Verification items for the finished model (mm, model axes). A direction names the side the tool comes from. Give positions to 0.01 mm unless a question says otherwise; leave off trailing zeros. Order: outer loops, then holes, each group sorted by start corner. A loop starts at its lowest first (then second) coordinate and runs counter-clockwise, first axis right, second up.
(1) Sectioned sample at C-C on x = 1.25. Record the cut outline in (y, z), plus the area to 3 significant figures.
(2) Gauge pin test, flat ends, axial feed: pin 1 (5 mm diameter, centred on x = 2, y = 0.5, fed in from -Z); pin 2 (2 mm diameter, centred on x = 8.5, z = 4.5, fed in from -Y); pin 3 (2 mm diameter, centred on x = 1.5, y = -10, fed in from +Z); pin 4 (7 mm diameter, centred on x = 0, y = 0, fed in from +Z). Record the tip position at first contact, or that the pin passes through.
(3) Sectioned sample at A-A on z = 5.5. Record the cut outline in (x, y), plus the area to 3 significant figures.
(4) Access from +Z, -Z, +X, -X, +Y, -Y to the whole of each face (thin tool, end or side, straight path). Record for faces 1 (the face through (-2, -9, 3)), 2 (the face through (-1.19, -5.37, 6.25)), 3 (the face through (4.71, 4.41, 2.96)).
(5) Sectioned sample at B-B on y = 8. Record the cut outline in (x, z).
(6) Scan lines: L1, parallel to Y at x = 0, z = 4.4; L2, parallel to Z at x = 0, y = -9.25; L3, parallel to Z at x = 1.5, y = -5.25. Record each from-to range of solid material in increasing order.
(7) Sectioned sample at D-D on z = 2.75. Record the cut outline in (x, y), plus the area to 3 significant figures.
(8) Mould release check, pull along X, two halves, no side actions. Record for faces 4 (the face through (0, 10, 3)), 5 (the face through (0.273, -14.998, 0.291)), 6 (the face through (-4.73, 4.29, 2.96)): pulls with the +X half, pulls with the -X half, needs draft (parallel to the pull), parting line crosses it, or undercut.
```python
from build123d import *

# Parameters (mm, degrees)
SKETCH1_R                           = 2
SKETCH1_R_2                         = 4
BOSS_EXTRUDE1_DEPTH                 = 6
SKETCH2_R                           = 5.5
SKETCH2_R_2                         = 4
BOSS_EXTRUDE2_DEPTH                 = 0.5
CUT_EXTRUDE1_REACH                  = 28.823
CUT_EXTRUDE1_END_RADIUS             = 15
CUT_EXTRUDE1_START                  = -5
SKETCH3_R                           = 2
CUT_EXTRUDE1_DIRECTION_2_REACH      = 28.823
CUT_EXTRUDE1_DIRECTION_2_END_RADIUS = 4


with BuildPart() as part:
    # Sketch1 → Boss-Extrude1 (new body)
    with BuildSketch(Plane.XY):
        with BuildLine():
            Line((5.5, 0), (14.456832295, -4))
            ThreePointArc((14.456832295, -4), (0, -15), (-14.456832295, -4))
            Line((-14.456832295, -4), (-5.5, 0))
            Line((-5.5, 0), (-3.937070517, 8.70673598))
            ThreePointArc((-3.937070517, 8.70673598), (0, 12), (3.937070517, 8.70673598))
            Line((3.937070517, 8.70673598), (5.5, 0))
        make_face()
        with Locations((0, 8)):
            Circle(SKETCH1_R, mode=Mode.SUBTRACT)
        Circle(SKETCH1_R_2, mode=Mode.SUBTRACT)
    extrude(amount=BOSS_EXTRUDE1_DEPTH)

    # Sketch2 → Boss-Extrude2 (add)
    with BuildSketch(Plane.XY.offset(6)):
        Circle(SKETCH2_R)
        Circle(SKETCH2_R_2, mode=Mode.SUBTRACT)
    extrude(amount=BOSS_EXTRUDE2_DEPTH)

    # Cut-Extrude1: up to this cylinder (the profile starts inside it)
    cut_extrude1_end = Plane(origin=(0, 0, 3), z_dir=(0, 0, -1)) * Cylinder(CUT_EXTRUDE1_END_RADIUS, 88.646, mode=Mode.PRIVATE)
    # Sketch3 → Cut-Extrude1 (cut, up to the surface)
    with BuildSketch(Plane(origin=(0, 0, 0), x_dir=(1, 0, 0), z_dir=(0, 1, 0)).offset(CUT_EXTRUDE1_START), mode=Mode.PRIVATE) as cut_extrude1_sk1:
        with Locations(Location((0, -3, 0), (0, 0, 270))):
            Circle(SKETCH3_R)
    cut_extrude1_tool1 = extrude(cut_extrude1_sk1.sketch, amount=-CUT_EXTRUDE1_REACH, mode=Mode.PRIVATE) & cut_extrude1_end
    add(cut_extrude1_tool1.solids().sort_by_distance((0, -5, 3))[0], mode=Mode.SUBTRACT)

    # Cut-Extrude1 direction 2: up to this cylinder (the profile starts outside it)
    cut_extrude1_direction_2_end = Plane(origin=(0, 0, 3), z_dir=(0, 0, -1)) * Cylinder(CUT_EXTRUDE1_DIRECTION_2_END_RADIUS, 66.646, mode=Mode.PRIVATE)
    # Sketch3 → Cut-Extrude1 direction 2 (cut, up to the surface)
    with BuildSketch(Plane(origin=(0, 0, 0), x_dir=(1, 0, 0), z_dir=(0, 1, 0)).offset(CUT_EXTRUDE1_START), mode=Mode.PRIVATE) as cut_extrude1_direction_2_sk1:
        with Locations(Location((0, -3, 0), (0, 0, 270))):
            Circle(SKETCH3_R)
    cut_extrude1_direction_2_tool1 = extrude(cut_extrude1_direction_2_sk1.sketch, amount=CUT_EXTRUDE1_DIRECTION_2_REACH, mode=Mode.PRIVATE) - cut_extrude1_direction_2_end
    add(cut_extrude1_direction_2_tool1.solids().sort_by_distance((0, -5, 3))[0], mode=Mode.SUBTRACT)


solid = part.part
```
Ans:
1. outline: (-14.95, 0) - (-3.8, 0) - (-3.8, 1.44) - (-14.95, 1.44) - close; (-14.95, 4.56) - (-3.8, 4.56) - (-3.8, 6.5) - (-5.36, 6.5) - (-5.36, 6) - (-14.95, 6) - close; (3.8, 0) - (6.44, 0) - (6.44, 6) - (5.36, 6) - (5.36, 6.5) - (3.8, 6.5) - close; (9.56, 0) - (11.8, 0) - (11.8, 6) - (9.56, 6) - close
1. area: 62.9 mm2
2. pin 1: stops at z = 0
2. pin 2: stops at y = -12.99
2. pin 3: stops at z = 6
2. pin 4: passes through
3. outline: (-14.46, -4) arc R15 ccw to (14.46, -4) - (5.5, 0) - (3.94, 8.71) arc R4 ccw to (-3.94, 8.71) - (-5.5, 0) - close; hole circle Ø8 at (0, 0); hole circle Ø4 at (0, 8)
3. area: 354 mm2
4. face 1: -Y
4. face 2: +Z
4. face 3: -Z, +X, +Y
5. outline: (-4.06, 0) - (-2, 0) - (-2, 6) - (-4.06, 6) - close; (2, 0) - (4.06, 0) - (4.06, 6) - (2, 6) - close
6. L1: y = 4 to 6, 10 to 12
6. L2: z = 0 to 1, 5 to 6
6. L3: z = 0 to 1.68, 4.32 to 6.5
7. outline: (-14.46, -4) arc R15 ccw to (-1.98, -14.87) - (-1.98, -3.47) arc R4 cw (long way) to (1.98, -3.47) - (1.98, -14.87) arc R15 ccw to (14.46, -4) - (5.5, 0) - (3.94, 8.71) arc R4 ccw to (-3.94, 8.71) - (-5.5, 0) - close; hole circle Ø4 at (0, 8)
7. area: 309 mm2
8. face 4: undercut
8. face 5: parting line crosses it
8. face 6: pulls with the -X half
